Model file for the job. Use its own axes, mm. A direction names the side the tool comes from. Coordinates: 2 decimals unless noted, no trailing zeros. Write each loop counter-clockwise with the first axis right and the second up, starting at its lowest first coordinate (ties: lowest second). Pieces come first, ordered by that corner, then holes. Notation, with made-up numbers: M -37.5,-8.75 L -7.5,-8.75 A31 ccw -7.5,18.25 Z; hole C 3,20 d8. An arc over 180 degrees is marked long. Put each result on its own line as item: value. Start each with the question number.
Q1. Cut at A-A (y = 10.5). Write the cut outline in (x, z), then the cut area to 3 significant figures.
Q2. Drill centre lines: line 1 along Z through (x, y) = (-20.5, 18.15); line 2 along X through (y, z) = (18.35, -28); line 3 along Z through (x, y) = (-32.15, 17.5). Where is each one in solid material? Low to high.
Q3. Cut at C-C (y = 17.5). Give the number of separate pieces and of enclosed holes in the cut face, then the cut area to 3 significant figures.
Q4. Cut at B-B (z = -19.5). Write the cut outline in (x, y).
Q5. Drop flat-ended pins along their axis: pin 1 (6.5 mm diameter, centred on y = 17.5, z = 36.6, fed in from -X); pin 2 (1.6 mm diameter, centred on x = -19, z = 27, fed in from +Y); pin 3 (3 mm diameter, centred on x = -13.5, y = 22.5, fed in from +Z); pin 4 (3 mm diameter, centred on x = 20, y = 24, fed in from +Z). Give the stop position or say it passes through.
Q6. Pull direction X, two halves, no side cores. Call faces 3 (the cylindrical face through (-33.63, 17.74, 39.65)), 4 (the cylindrical face through (-19.39, 19.36, 26.99)), 5 (the flat face through (0, 2.5, 36)), 6 (the flat face through (2, 4, 40)): pulls with the +X half, pulls with the -X half, needs draft (parallel to the pull), parting line crosses it, or undercut.
Q7. Which spindle directions (+Z, -Z, +X, -X, +Y, -Y) get a long thin tool onto all of the face, cutting with end or side? Do faces 1 (the cylindrical face through (33.7, 17.7, 39.6)), 2 (the flat face through (0, 20, -34)). Say none if no direction does.
Q8. Cut at D-D (x = 4). Write the cut outline in (y, z).
```python
from build123d import *

# Parameters (mm, degrees)
SKETCH1_W                                = 65
SKETCH1_H                                = 80
BOSS_EXTRUDE1_DEPTH                      = 5
SKETCH2_W                                = 65
SKETCH2_H                                = 80
SKETCH2_W_2                              = 57
SKETCH2_H_2                              = 68
BOSS_EXTRUDE2_DEPTH                      = 30
SKETCH3_R                                = 3.85
BOSS_EXTRUDE3_DEPTH                      = 20
F_3_0MM_DOWEL_HOLE1_D                    = 3
F_3_0MM_DOWEL_HOLE1_DEPTH                = 8.5
F_3_0MM_DOWEL_HOLE1_CSINK_D              = 3.05
F_3_0MM_DOWEL_HOLE1_CSINK_ANGLE          = 90
F_3_0MM_DOWEL_HOLE1_TIP                  = 0.901290929
CUT_EXTRUDE1_DEPTH                       = 2.7
MIRROR1_AT_THE_SECOND_PLANE_COPY_1_DEPTH = 2.7
SKETCH13_R                               = 2.75
CUT_EXTRUDE4_DEPTH                       = 2.4
SKETCH14_R                               = 1.5
CUT_EXTRUDE5_DEPTH                       = 4
SKETCH11_W                               = 57
SKETCH11_H                               = 6
CUT_EXTRUDE2_DEPTH                       = 30
SKETCH15_W                               = 57
SKETCH15_H                               = 3.1
CUT_EXTRUDE6_DEPTH                       = 2.5
SKETCH16_W                               = 80
SKETCH16_H                               = 35
SKETCH16_R                               = 2.75
BOSS_EXTRUDE4_DEPTH                      = 2
FILLET1_R                                = 2


with BuildPart() as part:
    # Sketch1 → Boss-Extrude1 (new body)
    with BuildSketch(Plane(origin=(0, 0, 0), x_dir=(1, 0, 0), z_dir=(0, 1, 0))):
        Rectangle(SKETCH1_W, SKETCH1_H)
    extrude(amount=BOSS_EXTRUDE1_DEPTH)

    # Sketch2 → Boss-Extrude2 (add)
    with BuildSketch(Plane(origin=(0, 5, 0), x_dir=(1, 0, 0), z_dir=(0, 1, 0))):
        Rectangle(SKETCH2_W, SKETCH2_H)
        Rectangle(SKETCH2_W_2, SKETCH2_H_2, mode=Mode.SUBTRACT)
    extrude(amount=BOSS_EXTRUDE2_DEPTH)

    # Sketch3 → Boss-Extrude3 (add)
    with BuildSketch(Plane(origin=(0, 5, 0), x_dir=(1, 0, 0), z_dir=(0, 1, 0))):
        with Locations(Location((-20.5, -28, 0), (0, 0, 90))):
            Circle(SKETCH3_R)
        with Locations(Location((20.5, -28, 0), (0, 0, 90))):
            Circle(SKETCH3_R)
        with Locations(Location((20.5, 28, 0), (0, 0, 90))):
            Circle(SKETCH3_R)
        with Locations(Location((-20.5, 28, 0), (0, 0, 90))):
            Circle(SKETCH3_R)
    extrude(amount=BOSS_EXTRUDE3_DEPTH)

    # Ø3.0mm Dowel Hole1
    with Locations(Plane(origin=(0, 25, 0), x_dir=(1, 0, 0), z_dir=(0, 1, 0))):
        with Locations((-20.5, 28), (20.5, 28), (20.5, -28), (-20.5, -28)):
            CounterSinkHole(F_3_0MM_DOWEL_HOLE1_D / 2, F_3_0MM_DOWEL_HOLE1_CSINK_D / 2, depth=F_3_0MM_DOWEL_HOLE1_DEPTH, counter_sink_angle=F_3_0MM_DOWEL_HOLE1_CSINK_ANGLE)
            with Locations((0, 0, -(F_3_0MM_DOWEL_HOLE1_DEPTH + F_3_0MM_DOWEL_HOLE1_TIP / 2))):  # 118° drill point
                Cone(0, F_3_0MM_DOWEL_HOLE1_D / 2, F_3_0MM_DOWEL_HOLE1_TIP, mode=Mode.SUBTRACT)

    # Sketch8 → Cut-Extrude1 (cut)
    with BuildSketch(Plane(origin=(0, 25, 0), x_dir=(1, 0, 0), z_dir=(0, 1, 0))):
        Polygon((-17.382308546, 28), (-18.941154273, 30.7), (-22.058845727, 30.7), (-23.617691454, 28), (-22.058845727, 25.3), (-18.941154273, 25.3), align=None)
    cut_extrude1 = extrude(amount=-CUT_EXTRUDE1_DEPTH, mode=Mode.SUBTRACT)

    # Mirror1: Cut-Extrude1 across plane
    add(cut_extrude1.mirror(Plane.XY), mode=Mode.SUBTRACT)

    # Mirror1 at the second plane: Cut-Extrude1 across plane
    add(cut_extrude1.mirror(Plane(origin=(0, 0, 0), x_dir=(0, 0, 1), z_dir=(1, 0, 0))), mode=Mode.SUBTRACT)

    # Mirror1 at the second plane copy 1 sketc → Mirror1 at the second plane copy 1 (cut)
    with BuildSketch(Plane(origin=(0, 25, 0), x_dir=(-1, 0, 0), z_dir=(0, 1, 0))):
        Polygon((-17.382308546, 28), (-18.941154273, 30.7), (-22.058845727, 30.7), (-23.617691454, 28), (-22.058845727, 25.3), (-18.941154273, 25.3), align=None)
    extrude(amount=-MIRROR1_AT_THE_SECOND_PLANE_COPY_1_DEPTH, mode=Mode.SUBTRACT)

    # Sketch13 → Cut-Extrude4 (cut)
    with BuildSketch(Plane(origin=(32.5, 0, 0), x_dir=(0, 0, -1), z_dir=(1, 0, 0))):
        with Locations((-36.6, 17.5)):
            Circle(SKETCH13_R)
    cut_extrude4 = extrude(amount=-CUT_EXTRUDE4_DEPTH, mode=Mode.SUBTRACT)

    # Sketch14 → Cut-Extrude5 (cut)
    with BuildSketch(Plane(origin=(32.5, 0, 0), x_dir=(0, 0, -1), z_dir=(1, 0, 0))):
        with Locations((-36.6, 17.5)):
            Circle(SKETCH14_R)
    cut_extrude5 = extrude(amount=-CUT_EXTRUDE5_DEPTH, mode=Mode.SUBTRACT)

    # Mirror2: Cut-Extrude4, Cut-Extrude5 across plane
    add(cut_extrude4.mirror(Plane(origin=(0, 0, 0), x_dir=(0, 0, 1), z_dir=(1, 0, 0))), mode=Mode.SUBTRACT)
    add(cut_extrude5.mirror(Plane(origin=(0, 0, 0), x_dir=(0, 0, 1), z_dir=(1, 0, 0))), mode=Mode.SUBTRACT)

    # Sketch11 → Cut-Extrude2 (cut)
    with BuildSketch(Plane(origin=(0, 35, 0), x_dir=(1, 0, 0), z_dir=(0, 1, 0))):
        with Locations((0, -37)):
            Rectangle(SKETCH11_W, SKETCH11_H)
    extrude(amount=-CUT_EXTRUDE2_DEPTH, mode=Mode.SUBTRACT)

    # Sketch15 → Cut-Extrude6 (cut)
    with BuildSketch(Plane(origin=(0, 5, 0), x_dir=(1, 0, 0), z_dir=(0, 1, 0))):
        with Locations((0, -35.55)):
            Rectangle(SKETCH15_W, SKETCH15_H)
    extrude(amount=-CUT_EXTRUDE6_DEPTH, mode=Mode.SUBTRACT)

    # Sketch16 → Boss-Extrude4 (add)
    with BuildSketch(Plane.ZY.offset(32.5)):
        with Locations((0, 17.5)):
            Rectangle(SKETCH16_W, SKETCH16_H)
        with Locations(Location((36.6, 17.5, 0), (0, 0, 180))):
            Circle(SKETCH16_R, mode=Mode.SUBTRACT)
    boss_extrude4 = extrude(amount=BOSS_EXTRUDE4_DEPTH)

    # Mirror3: Boss-Extrude4 across plane
    add(boss_extrude4.mirror(Plane(origin=(0, 0, 0), x_dir=(0, 0, 1), z_dir=(1, 0, 0))))

    # Fillet1
    # the kernel refuses this fillet: 2 mm, written as the material it takes off along each edge
    with BuildSketch(Plane(origin=(-34.5, -5, -40), x_dir=(1, 0, 0), z_dir=(0, 1, 0)), Plane(origin=(-34.5, 40, 40), x_dir=(1, 0, 0), z_dir=(0, -1, 0)), Plane(origin=(34.5, -5, -40), x_dir=(0, 0, 1), z_dir=(0, 1, 0))) as fillet1_piece_1:
        with BuildLine():
            CenterArc((FILLET1_R, -FILLET1_R), FILLET1_R, 90, 90)
            Line((0, -FILLET1_R), (0, 0))
            Line((0, 0), (FILLET1_R, 0))
        make_face()
    extrude(amount=45, mode=Mode.SUBTRACT)
    with BuildSketch(Plane(origin=(34.5, 40, 40), x_dir=(-1, 0, 0), z_dir=(0, -1, 0))) as fillet1_piece_2:
        with BuildLine():
            CenterArc((FILLET1_R, FILLET1_R), FILLET1_R, 180, 90)
            Line((0, FILLET1_R), (0, 0))
            Line((0, 0), (FILLET1_R, 0))
        make_face()
    extrude(amount=45, mode=Mode.SUBTRACT)


solid = part.part
```
Computed values:
1. outline: M -34.5,-38 A2 ccw -32.5,-40 L 32.5,-40 A2 ccw 34.5,-38 L 34.5,38 A2 ccw 32.5,40 L 28.5,40 L 28.5,-34 L -28.5,-34 L -28.5,40 L -32.5,40 A2 ccw -34.5,38 Z; C -20.5,-28 d7.7; C -20.5,28 d7.7; C 20.5,-28 d7.7; C 20.5,28 d7.7
1. area: 1,480 mm2
2. line 1: -40 to -34, -31.85 to -29.5, -26.5 to -24.15, 24.15 to 26.5, 29.5 to 31.85
2. line 2: -34.5 to -28.5, -24.35 to -22, -19 to -16.65, 16.65 to 19, 22 to 24.35, 28.5 to 34.5
2. line 3: -40 to 33.85, 39.35 to 40
3. separate pieces: 7
3. enclosed holes: 4
3. area: 1,400 mm2
4. outline: M -34.5,0 L 34.5,0 L 34.5,35 L 28.5,35 L 28.5,5 L -28.5,5 L -28.5,35 L -34.5,35 Z
5. pin 1: x = -34.5
5. pin 2: y = 22.3
5. pin 3: z = -34
5. pin 4: z = 31.85
6. face 3: pulls with the -X half
6. face 4: undercut
6. face 5: undercut
6. face 6: needs draft
7. face 1: +Z, +X, +Y, -Y
7. face 2: +Y
8. outline: M 0,-40 L 35,-40 L 35,-34 L 5,-34 L 5,34 L 2.5,34 L 2.5,37.1 L 5,37.1 L 5,40 L 0,40 Z
